```python
from build123d import *

# Parameters (mm, degrees)
SKETCH3_W                = 7.322640784
SKETCH3_H                = 100
BOSS_EXTRUDE1_DEPTH      = 80
FILLET1_R                = 60
FILLET2_R                = 20
FILLET3_R                = 20
FILLET4_R                = 20
CIRPATTERN2_COUNT        = 7
FILLET1_OF_CIRPATTERN2_R = 60
FILLET2_OF_CIRPATTERN2_R = 20
FILLET3_OF_CIRPATTERN2_R = 20
FILLET4_OF_CIRPATTERN2_R = 20


with BuildPart() as part:
    # Sketch2 → Revolve2 (revolve)
    with BuildSketch(Plane(origin=(0, 0, 0), x_dir=(0, 0, -1), z_dir=(1, 0, 0))):
        Polygon((32.860104606, 2), (10, 0), (10, 10), (60, 10), (60, 5), (175, 5), (175, 0), align=None)
    revolve(axis=Axis((0, 0, 0), (0, 1, 0)))

    # Sketch3 → Boss-Extrude1 (add)
    with BuildSketch(Plane(origin=(0, 5, 0), x_dir=(1, 0, 0), z_dir=(0, 1, 0))):
        with Locations((0, 145)):
            Rectangle(SKETCH3_W, SKETCH3_H)
    boss_extrude1 = extrude(amount=BOSS_EXTRUDE1_DEPTH)

    # Fillet1
    fillet1_edges = [part.edges().sort_by_distance(p)[0] for p in [
        (0, 85, -195),
    ]]
    fillet(fillet1_edges, radius=FILLET1_R)

    # Fillet2
    fillet2_edges = [part.edges().sort_by_distance(p)[0] for p in [
        (0, 5, -195),
    ]]
    fillet(fillet2_edges, radius=FILLET2_R - 0.0001)  # a hair under: the kernel refuses the full size

    # Fillet3
    fillet3_edges = [part.edges().sort_by_distance(p)[0] for p in [
        (0, 85, -95),
    ]]
    fillet(fillet3_edges, radius=FILLET3_R)

    # Fillet4
    fillet4_edges = [part.edges().sort_by_distance(p)[0] for p in [
        (0, 5, -95),
    ]]
    fillet(fillet4_edges, radius=FILLET4_R)

    # CirPattern2: Boss-Extrude1 ×7 about axis
    cirpattern2_axis = Axis((0, 0, 0), (0, 1, 0))
    for i in range(1, CIRPATTERN2_COUNT):
        add(boss_extrude1.rotate(cirpattern2_axis, i * 360 / CIRPATTERN2_COUNT))

    # Fillet1 of CirPattern2
    fillet1_of_cirpattern2_edges = [part.edges().sort_by_distance(p)[0] for p in [
        (-152.457139081, 85, -121.580511362),
        (-190.110942875, 85, 43.391582121),
        (-84.607329128, 85, 175.688929241),
        (84.607329128, 85, 175.688929241),
        (190.110942875, 85, 43.391582121),
        (152.457139081, 85, -121.580511362),
    ]]
    fillet(fillet1_of_cirpattern2_edges, radius=FILLET1_OF_CIRPATTERN2_R)

    # Fillet2 of CirPattern2
    fillet2_of_cirpattern2_edges = [part.edges().sort_by_distance(p)[0] for p in [
        (-152.457139081, 5, -121.580511362),
        (-190.110942875, 5, 43.391582121),
        (-84.607329128, 5, 175.688929241),
        (84.607329128, 5, 175.688929241),
        (190.110942875, 5, 43.391582121),
        (152.457139081, 5, -121.580511362),
    ]]
    fillet(fillet2_of_cirpattern2_edges, radius=FILLET2_OF_CIRPATTERN2_R - 0.0001)  # a hair under: the kernel refuses the full size

    # Fillet3 of CirPattern2
    fillet3_of_cirpattern2_edges = [part.edges().sort_by_distance(p)[0] for p in [
        (-74.273990834, 85, -59.231531177),
        (-92.618151657, 85, 21.139488726),
        (-41.218955216, 85, 85.592042451),
        (41.218955216, 85, 85.592042451),
        (92.618151657, 85, 21.139488726),
        (74.273990834, 85, -59.231531177),
    ]]
    fillet(fillet3_of_cirpattern2_edges, radius=FILLET3_OF_CIRPATTERN2_R)

    # Fillet4 of CirPattern2
    fillet4_of_cirpattern2_edges = [part.edges().sort_by_distance(p)[0] for p in [
        (-74.273990834, 5, -59.231531177),
        (-92.618151657, 5, 21.139488726),
        (-41.218955216, 5, 85.592042451),
        (41.218955216, 5, 85.592042451),
        (92.618151657, 5, 21.139488726),
        (74.273990834, 5, -59.231531177),
    ]]
    fillet(fillet4_of_cirpattern2_edges, radius=FILLET4_OF_CIRPATTERN2_R)


solid = part.part
```
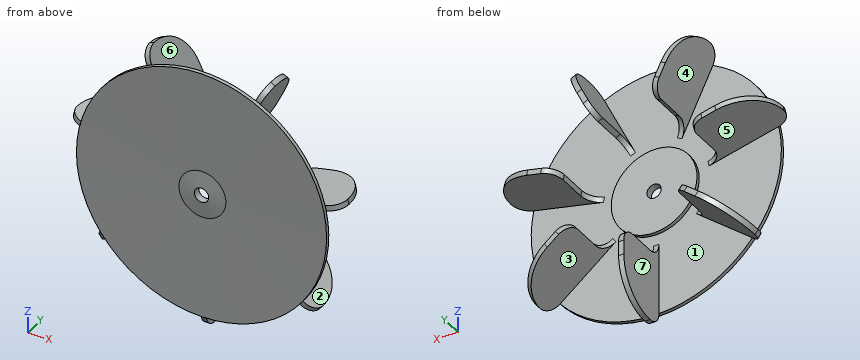
Work out the finished part from the listing and answer in its coordinate system (mm). Face numbers are marked on the shaded views. A direction names the side the tool comes from. Give positions to 0.01 mm unless a question says otherwise; leave off trailing zeros. Loops run counter-clockwise (first coordinate to the right, second up) from the corner with the lowest first, then second, coordinate; pieces in that order, holes last. Notation, with made-up numbers: (26.5, -6) - (68.5, -6) arc R8 ccw to (68.5, 0) - close; hole circle Ø10 at (45.5, 20.25). An arc over 180 degrees is marked (long way). One line per question, with ' | ' between items.
(1) The part is cut by section C-C (y = 77). Write down the section's boundary in (x, z), then the cut area to 3 significant figures.
Recorded:
outline: (-161.61, 33.13) - (-97.33, 18.46) - (-95.7, 25.6) - (-159.98, 40.27) - close; (-131.23, -99.97) - (-126.67, -105.7) - (-75.12, -64.59) - (-79.68, -58.86) - close; (-74.86, 147.01) - (-46.25, 87.61) - (-39.66, 90.78) - (-68.26, 150.19) - close; (-3.66, -164.93) - (3.66, -164.93) - (3.66, -99) - (-3.66, -99) - close; (39.66, 90.78) - (46.25, 87.61) - (74.86, 147.01) - (68.26, 150.19) - close; (75.12, -64.59) - (126.67, -105.7) - (131.23, -99.97) - (79.68, -58.86) - close; (95.7, 25.6) - (97.33, 18.46) - (161.61, 33.13) - (159.98, 40.27) - close | area: 3,380 mm²
(2) A tool of negligible diameter and unlimited length cuts with its end or side. For the marked faces 1, 2, 3 and 4, from which of +Z, -Z, +X, -X, +Y, -Y can it reach the whole face along a straight path? Write none if from no direction.
Recorded:
face 1: +Y | face 2: +X, +Y | face 3: -Z, +Y | face 4: -X, +Y
(3) Each of these flat-tipped pins is pushed along its axis until it touches: pin 1 Ø8 at (x, y) = (-94, 46) entering from -Z; pin 2 Ø1.5 at (x, y) = (-118.5, 56.5) entering from -Z; pin 3 Ø18 at (x, z) = (0, 0) entering from -Y; pin 4 Ø12 at (x, z) = (-70.5, -63) entering from +Y. Where does it stop, or does it pass through?
Recorded:
pin 1: stops at z = -82.84 | pin 2: stops at z = -99.78 | pin 3: passes through | pin 4: stops at y = 78.42
(4) The part is cut by section A-A (z = 0). Write down the section's boundary in (x, y), then the cut area to 3 significant figures.
Recorded:
outline: (-175, 0) - (-32.86, 2) - (-10, 0) - (-10, 10) - (-60, 10) - (-60, 5) - (-175, 5) - close; (10, 0) - (32.86, 2) - (175, 0) - (175, 5) - (60, 5) - (60, 10) - (10, 10) - close | area: 1,820 mm²
(5) Straight lines are drawn through the part: probe 1 along X at (y, z) = (6, 0); probe 2 along X at (y, z) = (22.5, -109); probe 3 along X at (y, z) = (5.5, -96). For each, find the intervals that lie inside material, in ascending order.
Recorded:
probe 1: x = -60 to -10, 10 to 60 | probe 2: x = -142.55 to -130.81, -3.66 to 3.66, 130.81 to 142.55 | probe 3: x = -126.25 to -114.51, -3.66 to 3.66, 114.51 to 126.25
(6) The mould has two halves that part along Z. Classify the marked faces 5, 6 and 7: +Z half, -Z half, draft (parallel to the pull), parting line (faces both ways), or undercut.
Recorded:
face 5: undercut | face 6: +Z half | face 7: draft
(7) The part is cut by section B-B (y = 56). Write down the section's boundary in (x, z).
Recorded:
outline: (-182.51, 37.9) - (-93.43, 17.57) - (-91.8, 24.71) - (-180.88, 45.04) - close; (-147.99, -113.34) - (-143.43, -119.06) - (-71.99, -62.09) - (-76.56, -56.37) - close; (-84.16, 166.33) - (-44.52, 84) - (-37.92, 87.18) - (-77.56, 169.5) - close; (-3.66, -186.37) - (3.66, -186.37) - (3.66, -95) - (-3.66, -95) - close; (37.92, 87.18) - (44.52, 84) - (84.16, 166.33) - (77.56, 169.5) - close; (71.99, -62.09) - (143.43, -119.06) - (147.99, -113.34) - (76.56, -56.37) - close; (91.8, 24.71) - (93.43, 17.57) - (182.51, 37.9) - (180.88, 45.04) - close
